Verification items for this drawing (mm, ordinates from the low corner). A direction names the side the tool comes from. Round coordinates to 2 decimals unless told otherwise and drop trailing zeros. Order: outer loops, then holes, each group sorted by start corner. A loop starts at its lowest first (then second) coordinate and runs counter-clockwise, first axis right, second up.
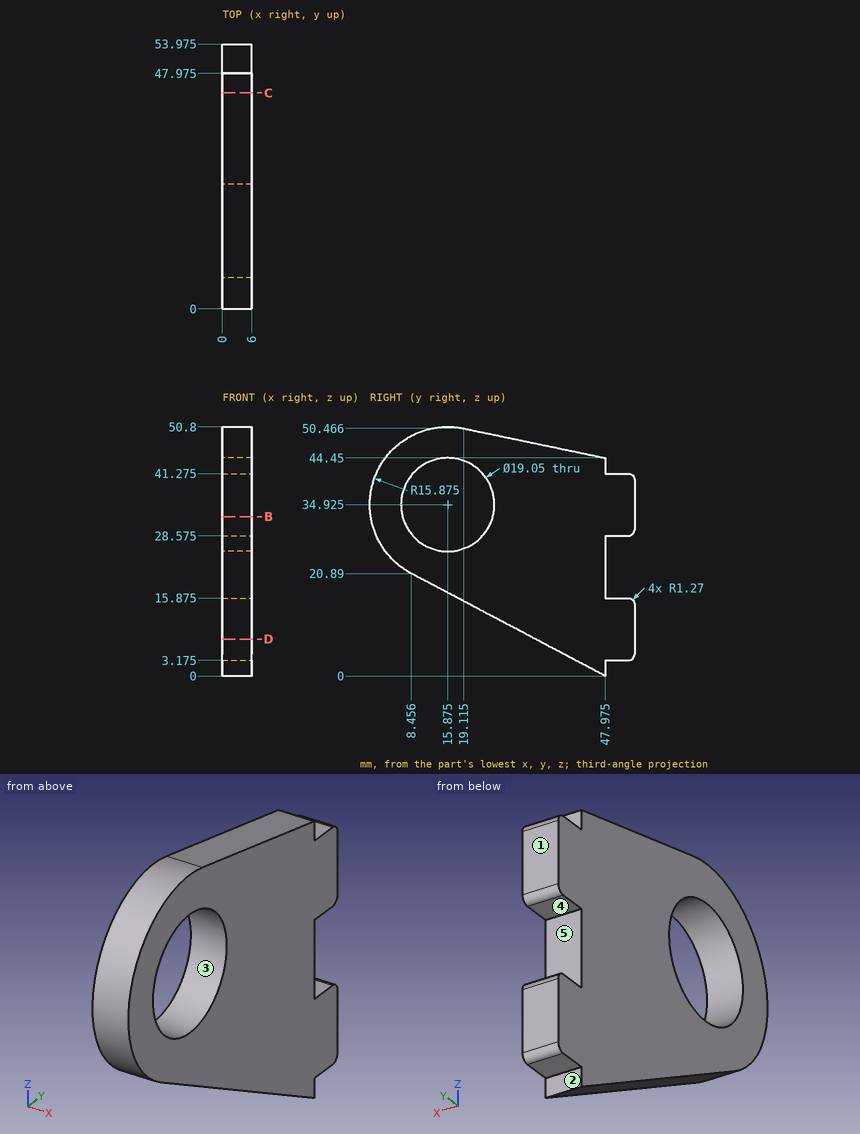
Item 1: Go/stop test with flat-tipped pins: P1, Ø1.6, axis at x = 3.5, z = 42.5, coming from the +Y side (1 decimal); P2, Ø2.5, axis at x = 3, y = 49.5, coming from the -Z side (1 decimal); P3, Ø2.5, axis at x = 2, y = 49.5, coming from the +Z side (1 decimal); P4, Ø11.5, axis at y = 15.875, z = 34.925, coming from the -X side. Record where each tip stops, or that it passes through.
Answer:
P1: stops at y = 48
P2: stops at z = 3.2
P3: stops at z = 41.3
P4: passes through
Item 2: Sectioned sample at C-C (y = 44). Record the cut outline in (x, z).
Answer:
outline: (0, 2.1) - (6, 2.1) - (6, 45.28) - (0, 45.28) - close
Item 3: Sectioned sample at B-B (z = 32.5). Record the cut outline in (x, y) (1 decimal).
Answer:
outline: (0, 0.2) - (6, 0.2) - (6, 6.7) - (0, 6.7) - close; (0, 25.1) - (6, 25.1) - (6, 54) - (0, 54) - close
Item 4: Sectioned sample at D-D (z = 7.5). Record the cut outline in (x, y) (1 decimal), and give its area (3 significant figures).
Answer:
outline: (0, 33.8) - (6, 33.8) - (6, 54) - (0, 54) - close
area: 121 mm2
Item 5: Scan lines: line 1 along Z through (x, y) = (3.85, 9) (1 decimal); line 2 along Z through (x, y) = (5.25, 7.5) (1 decimal); line 3 along Y through (x, z) = (3.65, 32) (1 decimal). Record each from-to range of solid material in increasing order.
Answer:
line 1: z = 20.6 to 28.3, 41.5 to 49.2
line 2: z = 21.4 to 30.4, 39.5 to 48.4
line 3: y = 0.3 to 6.8, 24.9 to 54
Item 6: Release check for a two-part mould opening along Y. For the marked faces 3, 4 and 5 record: released by +Y, released by -Y, zero draft, split by the parting line, or undercut.
Answer:
face 3: undercut
face 4: zero draft
face 5: released by +Y
Item 7: Access from +Z, -Z, +X, -X, +Y, -Y to the whole of each face (thin tool, end or side, straight path). Record for the marked faces 1 and 2.
Answer:
face 1: +Z, -Z, +X, -X, +Y
face 2: -Z, +X, -X, +Y
